Autodesk Inventor part; units mm, degrees
ref_plane "YZ Plane" through (0, 0, 0) normal (1, 0, 0) x (0, 1, 0)
ref_plane "XZ Plane" through (0, 0, 0) normal (0, 1, 0) x (-1, 0, 0)
ref_plane "XY Plane" through (0, 0, 0) normal (0, 0, 1) x (1, 0, 0)
sketch "Sketch1" plane through (0, 0, 0) normal (0, 1, 0) x (-1, 0, 0)
  circle A0 centre (0, 0) radius 3
  line L0 (12, 10) -> (-6, 10)
  line L1 (-10, 6) -> (-10, -5)
  line L2 (12, 10) -> (12, -1)
  line L3 (-10, -5) -> (8, -5)
  arc A1 (8, -5) -> (12, -1) centre (8, -1) ccw
  line L4 (-6, 10) -> (-10, 6)
  line L5 (-6, 10) -> (-0.3431, 10) construction
  line L6 (-6.4971, 11.2) -> (12, 11.2)
  line L7 (12, 11.2) -> (12, 10)
  line L8 (-10, -5) -> (-11.2, -5)
  line L9 (-11.2, -5) -> (-11.2, 6.4971)
  line L10 (-11.2, 6.4971) -> (-6.4971, 11.2)
  line L11 (12, 10) -> (12, 10)
  line L12 (-10, -5) -> (-10, -5)
  circle A2 centre (9, 0) radius 2
  point P0 (7, 0)
  dimension "d0" = 6
  dimension "d1" = 10
  dimension "d2" = 10
  dimension "d3" = 5
  dimension "d4" = 7
  dimension "d5" = 5
  dimension "d6" = 135
  dimension "d7" = 4
  dimension "d8" = 1.2
  dimension "d9" = 1.2
  dimension "d14" = 4
  dimension "d20" = 2
extrude "Extrusion1" add sketch "Sketch1" along normal blind 2 contours L2 A1 L3 L1 L4 L0 | L0 L4 L1 L8 L9 L10 L6 L7 | A2
extrude "Extrusion2" add sketch "Sketch1" against normal blind 4.6 contours L0 L4 L1 L8 L9 L10 L6 L7
extrude "Extrusion3" add sketch "Sketch1" along normal blind 14 contours A2
sketch "Sketch4" plane through (0, 0, 0) normal (0, -1, 0) x (1, 0, 0)
  circle A0 centre (0, 0) radius 3
  circle A1 centre (0, 0) radius 5.3
  circle A2 centre (0, 0) radius 3
  line L0 (10, -5) -> (-8, -5)
  point P0 (-1.7578, -5)
  point P1 (1.7578, -5)
  dimension "d23" = 10.6
extrude "Extrusion5" add sketch "Sketch4" along normal blind 4.6 contours A1 L0 picked at (-0.1205, -4.326)
ref_plane "Work Plane1" through (-7, 0, 0) normal (1, 0, 0) x (0, 1, 0)
sketch "Sketch5" plane through (-7, 0, 0) normal (1, 0, 0) x (0, 1, 0)
  circle A0 centre (12.5, 0) radius 0.75
  line L0 (2, 6.4971) -> (2, -5)
  point P0 (0, 0)
  dimension "d24" = 1.5
  dimension "d25" = 10.5
extrude "Extrusion6" cut sketch "Sketch5" against normal through all
fillet "Fillet1" radius 1 1 edges at (-7, 2, 0)
equation "\"d9\" = d8"
equation "\"sensorDistFromLens\" = 29"
equation "\"lensDistFromMetal\" = 12"
properties part number "stringHold"
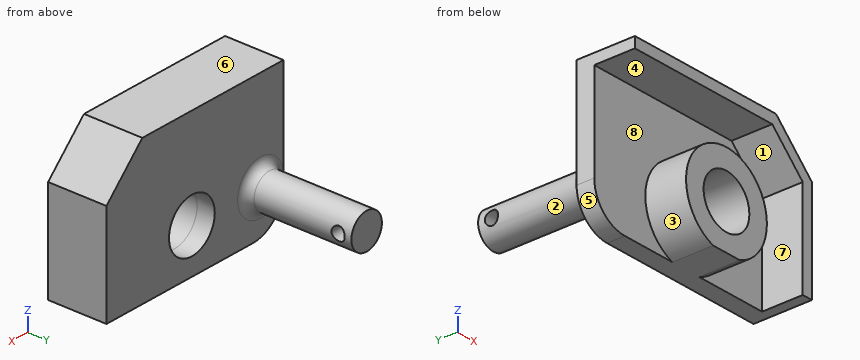
For this review, take the finished solid that the model builds, in its own axes (mm). Face numbers are marked on the shaded views. A direction names the side the tool comes from. Coordinates: 2 decimals unless noted, no trailing zeros. Loops run counter-clockwise (first coordinate to the right, second up) from the corner with the lowest first, then second, coordinate; pieces in that order, holes last. Notation, with made-up numbers: (66.5, -11) -> (100.5, -11) arc R17 ccw to (100.5, 5) -> close; hole circle Ø1 at (28, -4). An arc over 180 degrees is marked (long way). Return JSON: item names as keys, results as strings. Group by question number.
(1) Consider section B-B, the plane x = 0. Give the boundary of the cut face in (y, z), plus the area to 3 significant figures.
(2) Consider section D-D, the plane x = -9. Give the boundary of the cut face in (y, z).
(3) To check wall thickness, follow L1, parallel to X at y = -2.25, z = 0; L2, parallel to Z at x = 0, y = -1.5; L3, parallel to Y at x = -9.95, z = 0. State the ranges of each line that lie inside material, in increasing order.
(4) Mouldability with a two-part tool opening along X and no side actions: class the marked faces 5, 6, 7 and 8 as pulls with the +X half, pulls with the -X half, needs draft (parallel to the pull), parting line crosses it, or undercut.
(5) Tool access review of the marked faces 1, 2, 3 and 4: name each direction out of +Z, -Z, +X, -X, +Y, -Y from which nothing blocks a thin tool from reaching the whole face with its end or side.
(6) Consider section C-C, the plane y = -0.75. Give the boundary of the cut face in (x, z), plus the area to 3 significant figures.
(7) Consider section A-A, the plane z = 0. Count the separate pieces of the cut face and the enclosed holes in it, plus the area to 3 significant figures.
(8) For pin 1 Ø8 at (y, z) = (3, 9.5) entering from +X; pin 2 Ø1.4 at (y, z) = (-1.5, 2) entering from -X; pin 3 Ø1 at (y, z) = (-1.5, -2.5) entering from -X; pin 4 Ø2 at (y, z) = (5.5, 0) entering from -X, all flat-tipped, find the tip position at first contact; note any pin that passes through.
Results below:
{
 "1": {"outline": "(-4.6, -5) -> (2, -5) -> (2, -3) -> (-4.6, -3) -> close; (-4.6, 3) -> (2, 3) -> (2, 11.2) -> (-4.6, 11.2) -> (-4.6, 10) -> (0, 10) -> (0, 5.3) -> (-4.6, 5.3) -> close", "area": "45.7 mm2"},
 "2": {"outline": "(-4.6, 10) -> (0, 10) -> (0, -4.87) -> (2, -4.87) -> (2, -3) arc R1 cw to (3, -2) -> (14, -2) -> (14, 2) -> (3, 2) arc R1 cw to (2, 3) -> (2, 11.2) -> (-4.6, 11.2) -> close; hole circle Ø1.5 at (12.5, 0)"},
 "3": {"L1": "x = -5.3 to -3, 3 to 5.3, 10 to 11.2", "L2": "z = -5 to -3, 3 to 5.3, 10 to 11.2", "L3": "y = 0 to 11.75, 13.25 to 14"},
 "4": {"face 5": "pulls with the -X half", "face 6": "needs draft", "face 7": "undercut", "face 8": "undercut"},
 "5": {"face 1": "-Z, -X, -Y", "face 2": "+Y", "face 3": "-Y", "face 4": "-X, -Y"},
 "6": {"outline": "(-12, 10) -> (6, 10) -> (10, 6) -> (10, -5) -> (11.2, -5) -> (11.2, 6.5) -> (6.5, 11.2) -> (-12, 11.2) -> close; (-1.76, -5) -> (1.76, -5) arc R5.3 ccw (long way) to start; hole circle Ø6 at (0, 0)", "area": "102 mm2"},
 "7": {"separate pieces": "3", "enclosed holes": "0", "area": "104 mm2"},
 "8": {"pin 1": "stops at x = 11.2", "pin 2": "stops at x = -5.14", "pin 3": "stops at x = -4.91", "pin 4": "stops at x = -11"}
}
